```python
from build123d import *

# Parameters (mm, degrees)
SKETCH_1_W      = 59
SKETCH_1_H      = 23
EXTRUDE_1_DEPTH = 49
EXTRUDE_START   = -11
EXTRUDE_2_DEPTH = 30
EXTRUDE_3_DEPTH = 0.6


with BuildPart() as part:
    # 草图1 → 拉伸1 (new body)
    with BuildSketch(Plane.XY):
        Rectangle(SKETCH_1_W, SKETCH_1_H)
    extrude(amount=EXTRUDE_1_DEPTH)

    # 草图2 → 拉伸2 (add)
    with BuildSketch(Plane.XY.offset(49).offset(EXTRUDE_START)):
        with BuildLine():
            Line((-8.5, 22.5), (8.5, 22.5))
            ThreePointArc((8.5, 22.5), (15.571067812, 19.571067812), (18.5, 12.5))
            Line((18.5, 12.5), (18.5, -12.5))
            ThreePointArc((18.5, -12.5), (15.571067812, -19.571067812), (8.5, -22.5))
            Line((8.5, -22.5), (-8.5, -22.5))
            ThreePointArc((-8.5, -22.5), (-15.571067812, -19.571067812), (-18.5, -12.5))
            Line((-18.5, -12.5), (-18.5, 12.5))
            ThreePointArc((-18.5, 12.5), (-15.571067812, 19.571067812), (-8.5, 22.5))
        make_face()
    extrude(amount=-EXTRUDE_2_DEPTH)

    # 草图3 → 拉伸3 (add)
    # profile 1 of 2: a face of its own
    with BuildSketch(Plane(origin=(0, 0, 0), x_dir=(-1, 0, 0), z_dir=(0, 0, -1))):
        with BuildLine():
            Line((-29.5, 7.5), (-36.5, 7.5))
            ThreePointArc((-36.5, 7.5), (-40.035533906, 6.035533906), (-41.5, 2.5))
            Line((-41.5, 2.5), (-41.5, -2.5))
            ThreePointArc((-41.5, -2.5), (-40.035533906, -6.035533906), (-36.5, -7.5))
            Line((-36.5, -7.5), (-29.5, -7.5))
            Line((-29.5, -7.5), (-29.5, 7.5))
        make_face()
        with BuildLine():
            Line((-36.75, 2.25), (-34.75, 2.25))
            ThreePointArc((-34.75, 2.25), (-32.5, 0), (-34.75, -2.25))
            Line((-34.75, -2.25), (-36.75, -2.25))
            ThreePointArc((-36.75, -2.25), (-39, 0), (-36.75, 2.25))
        make_face(mode=Mode.SUBTRACT)
    # profile 2 of 2: a face of its own
    with BuildSketch(Plane(origin=(0, 0, 0), x_dir=(-1, 0, 0), z_dir=(0, 0, -1))):
        with BuildLine():
            Line((41.5, 2.5), (41.5, -2.5))
            ThreePointArc((41.5, -2.5), (40.035533906, -6.035533906), (36.5, -7.5))
            Line((36.5, -7.5), (29.5, -7.5))
            Line((29.5, -7.5), (29.5, 7.5))
            Line((29.5, 7.5), (36.5, 7.5))
            ThreePointArc((36.5, 7.5), (40.035533906, 6.035533906), (41.5, 2.5))
        make_face()
        with BuildLine():
            Line((36.75, 2.25), (34.75, 2.25))
            ThreePointArc((34.75, 2.25), (32.5, 0), (34.75, -2.25))
            Line((34.75, -2.25), (36.75, -2.25))
            ThreePointArc((36.75, -2.25), (39, 0), (36.75, 2.25))
        make_face(mode=Mode.SUBTRACT)
    extrude(amount=-EXTRUDE_3_DEPTH)


solid = part.part
```
Model file for the job. Use its own axes, mm. A direction names the side the tool comes from. Give positions to 0.01 mm unless a question says otherwise; leave off trailing zeros. Order: outer loops, then holes, each group sorted by start corner. A loop starts at its lowest first (then second) coordinate and runs counter-clockwise, first axis right, second up.
1) 3-axis set-ups, long thin cutter, end or side, ignore diameter. For faces 5 (the cylindrical face through (32.5, 0, 0.3)), 6 (the flat face through (0, -22.5, 23)), 7 (the flat face through (-33, 2, 0.6)), 8 (the flat face through (0, 17, 38)): which of +Z, -Z, +X, -X, +Y, -Y reach the whole face in a straight line?
2) Wall check: probe 1 along Z at (x, y) = (-14, -14); probe 2 along Z at (x, y) = (37.5, 5); probe 3 along Y at (x, z) = (26.5, 4). Give the ranges that are in metal, low to high.
3) Saw through at B-B, the plane x = 6.5. Write the cut outline in (y, z), then the cut area to 3 significant figures.
4) Saw through at C-C, the plane z = 37. Write the cut outline in (x, y).
5) Pin check, flat tips, straight feed: pin 1 (13 mm diameter, centred on x = 37, y = 0, fed in from +Z); pin 2 (0.5 mm diameter, centred on x = -33, z = 0.5, fed in from -Y); pin 3 (12 mm diameter, centred on y = 4.5, z = 23.5, fed in from -X). Stop position of each tip, or through.
6) Saw through at D-D, the plane y = -10.5. Write the cut outline in (x, z), then the cut area to 3 significant figures.
7) Mould opens along Y. For faces 1 (the cylindrical face through (39, 0, 0.3)), 2 (the cylindrical face through (40.07, -6, 0.3)), 3 (the flat face through (0, 17, 8)), 4 (the flat face through (0, 22.5, 23)) say: +Y half, -Y half, draft (parallel to the pull), parting line (faces both ways), or undercut.
8) Saw through at A-A, the plane y = 0. Write the cut outline in (x, z), then the cut area to 3 significant figures.
Computed:
1. face 5: +Z, -Z
1. face 6: +Z, -Z, +X, -X, -Y
1. face 7: +Z, -X, +Y, -Y
1. face 8: +Z, +X, -X, +Y
2. probe 1: z = 8 to 38
2. probe 2: z = 0 to 0.6
2. probe 3: y = -11.5 to 11.5
3. outline: (-22.5, 8) - (-11.5, 8) - (-11.5, 0) - (11.5, 0) - (11.5, 8) - (22.5, 8) - (22.5, 38) - (11.5, 38) - (11.5, 49) - (-11.5, 49) - (-11.5, 38) - (-22.5, 38) - close
3. area: 1,790 mm2
4. outline: (-29.5, -11.5) - (-18.5, -11.5) - (-18.5, -12.5) arc R10 ccw to (-8.5, -22.5) - (8.5, -22.5) arc R10 ccw to (18.5, -12.5) - (18.5, -11.5) - (29.5, -11.5) - (29.5, 11.5) - (18.5, 11.5) - (18.5, 12.5) arc R10 ccw to (8.5, 22.5) - (-8.5, 22.5) arc R10 ccw to (-18.5, 12.5) - (-18.5, 11.5) - (-29.5, 11.5) - close
5. pin 1: stops at z = 0.6
5. pin 2: stops at y = -7.5
5. pin 3: stops at x = -29.5
6. outline: (-29.5, 0) - (29.5, 0) - (29.5, 49) - (-29.5, 49) - close
6. area: 2,890 mm2
7. face 1: undercut
7. face 2: -Y half
7. face 3: draft
7. face 4: +Y half
8. outline: (-41.5, 0) - (-39, 0) - (-39, 0.6) - (-41.5, 0.6) - close; (-32.5, 0) - (32.5, 0) - (32.5, 0.6) - (29.5, 0.6) - (29.5, 49) - (-29.5, 49) - (-29.5, 0.6) - (-32.5, 0.6) - close; (39, 0) - (41.5, 0) - (41.5, 0.6) - (39, 0.6) - close
8. area: 2,900 mm2
